from build123d import *

# Parameters (mm, degrees)
SKETCH1_W           = 4
SKETCH1_H           = 20
BOSS_EXTRUDE1_DEPTH = 100


with BuildPart() as part:
    # Sketch1 → Boss-Extrude1 (new body)
    with BuildSketch(Plane.XY):
        Polygon((-12.5, 15), (-12.5, 10), (-2, 10), (2, 10), (12.5, 10), (12.5, 15), align=None)
        Rectangle(SKETCH1_W, SKETCH1_H)
        Polygon((-12.5, -10), (-12.5, -15), (12.5, -15), (12.5, -10), (2, -10), (-2, -10), align=None)
    extrude(amount=-BOSS_EXTRUDE1_DEPTH)


solid = part.part
Can you work these out from the model? Positions are in its coordinate system, mm. A direction names the side the tool comes from. Round coordinates to 2 decimals unless told otherwise and drop trailing zeros. Order: outer loops, then holes, each group sorted by start corner. A loop starts at its lowest first (then second) coordinate and runs counter-clockwise, first axis right, second up. Notation, with made-up numbers: (46, -22.75) -> (89, -22.75) arc R22 cw to (89, -0.75) -> close; hole circle Ø5 at (46, 21.5). An arc over 180 degrees is marked (long way). Write each question's results on one line, items separated by ' | '. Start each with the question number.
Item 1: If we section it at A-A, the plane x = -7.5: Write out the boundary of the cut face in (y, z), then the cut area to 3 significant figures.
Item 2: Will these pins go through, and if not, where does the flat tip stop? pin 1 (6 mm diameter, centred on y = -1.5, z = -41.5, fed in from -X); pin 2 (6 mm diameter, centred on y = 1.5, z = -35.5, fed in from +X).
Item 3: If we section it at B-B, the plane z = -36: Write out the boundary of the cut face in (x, y).
Item 4: Which directions (+Z, -Z, +X, -X, +Y, -Y) give clear straight access to the entire face, cutting with the end or side of a thin tool? Please do faces 1 (the flat face through (7, 10, -49)), 2 (the flat face through (0, 4, 0)), 3 (the flat face through (-7, -10, -49)).
Item 5: If we section it at C-C, the plane y = -5.25: Write out the boundary of the cut face in (x, z).
Item 6: Please list where these lines run through material, in increasing order: L1, parallel to Y at x = 8.75, z = -66; L2, parallel to X at y = -9.25, z = -7.
Results:
1) outline: (-15, -100) -> (-10, -100) -> (-10, 0) -> (-15, 0) -> close; (10, -100) -> (15, -100) -> (15, 0) -> (10, 0) -> close | area: 1,000 mm2
2) pin 1: stops at x = -2 | pin 2: stops at x = 2
3) outline: (-12.5, -15) -> (12.5, -15) -> (12.5, -10) -> (2, -10) -> (2, 10) -> (12.5, 10) -> (12.5, 15) -> (-12.5, 15) -> (-12.5, 10) -> (-2, 10) -> (-2, -10) -> (-12.5, -10) -> close
4) face 1: +Z, -Z, +X | face 2: +Z, +X, -X, +Y, -Y | face 3: +Z, -Z, -X
5) outline: (-2, -100) -> (2, -100) -> (2, 0) -> (-2, 0) -> close
6) L1: y = -15 to -10, 10 to 15 | L2: x = -2 to 2
